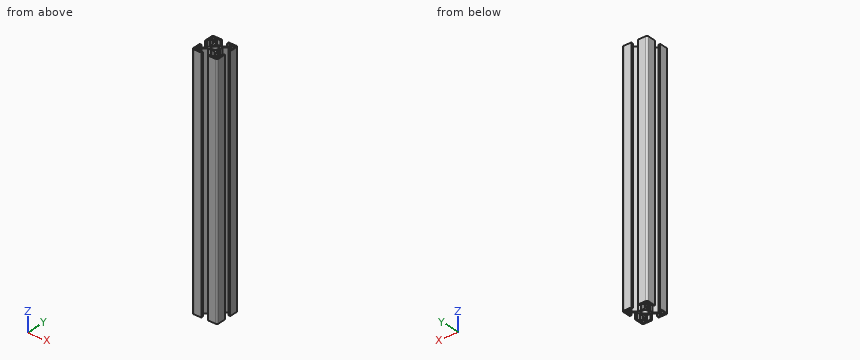
Autodesk Inventor part; units mm, degrees
ref_plane "YZ Plane" through (0, 0, 0) normal (1, 0, 0) x (0, 1, 0)
ref_plane "XZ Plane" through (0, 0, 0) normal (0, 1, 0) x (-1, 0, 0)
ref_plane "XY Plane" through (0, 0, 0) normal (0, 0, 1) x (1, 0, 0)
sketch "Náčrt1" plane through (0, 0, 0) normal (0, 0, 1) x (1, 0, 0)
  line L0 (0, -21.5799) -> (0, 21.5799)
  line L1 (-21.5799, 0) -> (21.5799, 0)
  line L2 (-13, 15) -> (-4, 15)
  line L3 (-4, 15) -> (-4, 13)
  line L4 (-4, 13) -> (-8.25, 13)
  line L5 (-8.25, 13) -> (-8.25, 9.6642)
  line L6 (-8.25, 9.6642) -> (-4, 5.4142)
  line L7 (-4, 5.4142) -> (-0.5196, 5.4142)
  line L8 (-0.5196, 5.4142) -> (0, 5.1142)
  line L9 (0, 5.1142) -> (0.5196, 5.4142)
  line L10 (0.5196, 5.4142) -> (4, 5.4142)
  line L11 (4, 5.4142) -> (8.25, 9.6642)
  line L12 (8.25, 9.6642) -> (8.25, 13)
  line L13 (8.25, 13) -> (4, 13)
  line L14 (4, 13) -> (4, 15)
  line L15 (4, 15) -> (13, 15)
  line L16 (15, 13) -> (15, 4)
  line L17 (15, 4) -> (13, 4)
  line L18 (13, 4) -> (13, 8.25)
  line L19 (13, 8.25) -> (9.6642, 8.25)
  line L20 (9.6642, 8.25) -> (5.4142, 4)
  line L21 (5.4142, 4) -> (5.4142, 0.5196)
  line L22 (5.4142, 0.5196) -> (5.1142, 0)
  line L23 (5.1142, 0) -> (5.4142, -0.5196)
  line L24 (5.4142, -0.5196) -> (5.4142, -4)
  line L25 (5.4142, -4) -> (9.6642, -8.25)
  line L26 (9.6642, -8.25) -> (13, -8.25)
  line L27 (13, -8.25) -> (13, -4)
  line L28 (13, -4) -> (15, -4)
  line L29 (15, -4) -> (15, -13)
  line L30 (13, -15) -> (4, -15)
  line L31 (-15, 13) -> (-15, 4)
  line L32 (-15, 4) -> (-13, 4)
  line L33 (-13, 4) -> (-13, 8.25)
  line L34 (-13, 8.25) -> (-9.6642, 8.25)
  line L35 (-9.6642, 8.25) -> (-5.4142, 4)
  line L36 (-5.4142, 4) -> (-5.4142, 0.5196)
  line L37 (-5.4142, 0.5196) -> (-5.1142, 0)
  line L38 (-5.1142, 0) -> (-5.4142, -0.5196)
  line L39 (-5.4142, -0.5196) -> (-5.4142, -4)
  line L40 (-5.4142, -4) -> (-9.6642, -8.25)
  line L41 (-9.6642, -8.25) -> (-13, -8.25)
  line L42 (-13, -8.25) -> (-13, -4)
  line L43 (-13, -4) -> (-15, -4)
  line L44 (-15, -4) -> (-15, -13)
  line L45 (-13, -15) -> (-4, -15)
  line L46 (-4, -15) -> (-4, -13)
  line L47 (-8.25, -9.6642) -> (-4, -5.4142)
  line L48 (-4, -5.4142) -> (-0.5196, -5.4142)
  line L49 (-0.5196, -5.4142) -> (0, -5.1142)
  line L50 (0, -5.1142) -> (0.5196, -5.4142)
  line L51 (0.5196, -5.4142) -> (4, -5.4142)
  line L52 (4, -5.4142) -> (8.25, -9.6642)
  line L53 (8.25, -9.6642) -> (8.25, -13)
  line L54 (8.25, -13) -> (4, -13)
  line L55 (4, -13) -> (4, -15)
  line L56 (-4, -13) -> (-8.25, -13)
  line L57 (-8.25, -13) -> (-8.25, -9.6642)
  circle A0 centre (-11.625, 11.625) radius 2.1
  circle A1 centre (11.625, 11.625) radius 2.1
  circle A2 centre (11.625, -11.625) radius 2.1
  circle A3 centre (-11.625, -11.625) radius 2.1
  circle A4 centre (0, 0) radius 3.4
  arc A5 (-13, 15) -> (-15, 13) centre (-13, 13) ccw
  arc A6 (15, 13) -> (13, 15) centre (13, 13) ccw
  arc A7 (13, -15) -> (15, -13) centre (13, -13) ccw
  arc A8 (-15, -13) -> (-13, -15) centre (-13, -13) ccw
  line L58 (-5.1142, 0) -> (-3.4, 0)
  line L59 (0, -5.1142) -> (0, -3.4)
  line L60 (5.1142, 0) -> (3.4, 0)
  line L61 (0, 5.1142) -> (0, 3.4)
  point P0 (15, -15)
  dimension "d0" = 120
  dimension "d1" = 0.3
  dimension "d2" = 30
  dimension "d3" = 8
  dimension "d4" = 2
  dimension "d5" = 6.75
  dimension "d6" = 120
  dimension "d7" = 2
  dimension "d8" = 4.2
  dimension "d9" = 23.25
  dimension "d10" = 23.25
  dimension "d11" = 6.8
  dimension "d12" = 2
extrude "Vysunutí1" add sketch "Náčrt1" along normal blind 289 contours L49 L48 L47 L57 L56 L46 L45 A8 L44 L43 L42 L41 L40 L39 L38 L1 A4 L0 | L0 A4 L1 L23 L24 L25 L26 L27 L28 L29 A7 L30 L55 L54 L53 L52 L51 L50 | L1 L37 L36 L35 L34 L33 L32 L31 A5 L2 L3 L4 L5 L6 L7 L8 L0 A4 | A4 L0 L9 L10 L11 L12 L13 L14 L15 A6 L16 L17 L18 L19 L20 L21 L22 L1
thread "Závit1"
thread "Závit2"
thread "Závit3"
thread "Závit4"
chamfer "Zkosení1" distance 0.75 angle 45 4 edges at (9.525, 11.625, 0) (-13.725, -11.625, 0) (-13.725, -11.625, 289) (9.525, 11.625, 289)
thread "Závit5"
thread "Závit6"
thread "Závit7"
thread "Závit8"
chamfer "Zkosení2" distance 0.75 angle 45 4 edges at (-13.725, 11.625, 289) (9.525, -11.625, 289) (9.525, -11.625, 0) (-13.725, 11.625, 0)
chamfer "Zkosení3" distance 0.75 angle 45 2 edges at (0, -3.4, 289) (0, -3.4, 0)
equation "\"d6\" = d0"
equation "\"d7\" = d4"
Could you check a few things on this model? Use its own coordinates, in mm. Round coordinates to 2 decimals unless told otherwise and drop trailing zeros. Write each question's results on one line, items separated by ' | '. Start each with the question number.
1. I need wall thicknesses on L1, parallel to Y at x = 12, z = 89; L2, parallel to Y at x = 6.25, z = 41; L3, parallel to X at y = 0, z = 230.5. Which ranges of each line are inside material? Lowest first, please. Write a range as from..to.
2. Imagine slicing it at A-A on z = 81.5. Count the separate pieces of the cut face and the enclosed holes in it, and give its area (3 significant figures).
3. I'm going to push flat-ended pins straight in: pin 1 Ø0.6 at (x, z) = (-14, 141.5) entering from -Y; pin 2 Ø1 at (x, z) = (2, 124) entering from +Y; pin 3 Ø2 at (y, z) = (-1.5, 172.5) entering from -X. Where does each tip first touch, or does it pass through?
Result sheet:
1) L1: y = -15..-13.69, -9.56..-8.25, 8.25..9.56, 13.69..15 | L2: y = -15..-13, -7.66..-4.84, 4.84..7.66, 13..15 | L3: x = -5.11..-3.4, 3.4..5.11
2) separate pieces: 1 | enclosed holes: 5 | area: 312 mm^2
3) pin 1: stops at y = -14.87 | pin 2: stops at y = 5.41 | pin 3: stops at x = -5.41
